Can you work these out from the model? Positions are in its coordinate system, mm. A direction names the side the tool comes from. Give positions to 0.01 mm unless a question says otherwise; leave off trailing zeros. Write each loop counter-clockwise with the first axis right and the second up, starting at its lowest first coordinate (ties: lowest second). Pieces come first, ordered by that corner, then holes. Notation, with made-up numbers: (5, 66.5) -> (58, 66.5) arc R24 ccw to (58, 92.5) -> close; hole circle Ø7 at (32, 82). An arc over 180 degrees is marked (long way). Answer as CSV lines item,"result". Start each with the question number.
1. If we section it at D-D on x = -8.5: Write out the boundary of the cut face in (y, z), plus the area to 3 significant figures.
2. I need wall thicknesses on line 1 (Z direction, x = -25.5, y = 0); line 2 (Z direction, x = 3.5, y = 0); line 3 (X direction, y = -1, z = -8). Which ranges of each line are inside material? Lowest first, please. Write a range as [from, to].
3. On a 3-axis mill with a long thin cutter (end or side, diameter ignored), from which of +Z, -Z, +X, -X, +Y, -Y can I reach the whole of each face in a straight line? I mean faces 1 (the face through (15.1, -1.5, 11.4)), 2 (the face through (-24.93, -4.38, -8.43)), 3 (the face through (0.1, 12.5, -0.1)). Say none if no direction works.
4. If we section it at C-C on x = 1: Write out the boundary of the cut face in (y, z), plus the area to 3 significant figures.
5. I'm going to push flat-ended pins straight in: P1, Ø3, axis at x = 11, z = 3.5, coming from the -Y side; P2, Ø12, axis at y = 0, z = 0, coming from the -X side; P3, Ø5, axis at x = 13.5, z = 9, coming from the -Y side; P4, Ø3, axis at x = -16.5, z = -3, coming from the +Y side. Where does each tip first touch, or does it pass through?
6. If we section it at B-B on y = 0: Write out the boundary of the cut face in (x, z), plus the area to 3 significant figures.
7. If we mould it in two halves opening along Y, with no side actions, what happens to faces 4 (the face through (10, -5, -11)), 5 (the face through (0.1, -12.5, 0.1)), 6 (the face through (0.14, 12.534, -7.29)), 7 (the face through (0.1, 0, 14.5))? For each: pulls with the +Y half, pulls with the -Y half, needs draft (parallel to the pull), parting line crosses it, or undercut.
8. If we section it at A-A on z = 0: Write out the boundary of the cut face in (x, y).
```python
from build123d import *

# Parameters (mm, degrees)
F0_R     = 8.5
F1_DEPTH = 10
F2_R     = 11.5
F2_R_2   = 8.5
F3_DEPTH = 20
F4_R     = 9.5
F4_R_2   = 7.5
F5_DEPTH = 10
F6_R     = 9.5
F7_DEPTH = 25


with BuildPart() as f1:
    # F0 (on Right) → F1 (new body, symmetric)
    with BuildSketch(Plane.YZ):
        with BuildLine():
            ThreePointArc((11.6835483463, -4.4435006516), (12.2941928228, -2.2589428581), (12.5, 0))
            ThreePointArc((12.5, 0), (12.2941928228, 2.2589428581), (11.6835483463, 4.4435006516))
            ThreePointArc((11.6835483463, 4.4435006516), (10.8253175473, 6.25), (9.6899586191, 7.8964993484))
            ThreePointArc((9.6899586191, 7.8964993484), (6.25, 10.8253175473), (1.9935897271, 12.34))
            ThreePointArc((1.9935897271, 12.34), (0, 12.5), (-1.9935897271, 12.34))
            ThreePointArc((-1.9935897271, 12.34), (-6.25, 10.8253175473), (-9.6899586191, 7.8964993484))
            ThreePointArc((-9.6899586191, 7.8964993484), (-10.8253175473, 6.25), (-11.6835483463, 4.4435006516))
            ThreePointArc((-11.6835483463, 4.4435006516), (-12.5, 0), (-11.6835483463, -4.4435006516))
            ThreePointArc((-11.6835483463, -4.4435006516), (-10.8253175473, -6.25), (-9.6899586191, -7.8964993484))
            ThreePointArc((-9.6899586191, -7.8964993484), (-6.25, -10.8253175473), (-1.9935897271, -12.34))
            ThreePointArc((-1.9935897271, -12.34), (0, -12.5), (1.9935897271, -12.34))
            ThreePointArc((1.9935897271, -12.34), (6.25, -10.8253175473), (9.6899586191, -7.8964993484))
            ThreePointArc((9.6899586191, -7.8964993484), (10.8253175473, -6.25), (11.6835483463, -4.4435006516))
        make_face()
        Circle(F0_R, mode=Mode.SUBTRACT)
        with BuildLine():
            ThreePointArc((9.6899586191, 7.8964993484), (10.8253175473, 6.25), (11.6835483463, 4.4435006516))
            ThreePointArc((11.6835483463, 4.4435006516), (12.5573683549, 7.25), (9.6899586191, 7.8964993484))
        make_face()
        with BuildLine():
            ThreePointArc((9.6899586191, -7.8964993484), (12.5573683549, -7.25), (11.6835483463, -4.4435006516))
            ThreePointArc((11.6835483463, -4.4435006516), (10.8253175473, -6.25), (9.6899586191, -7.8964993484))
        make_face()
        with BuildLine():
            ThreePointArc((-1.9935897271, 12.34), (0, 12.5), (1.9935897271, 12.34))
            ThreePointArc((1.9935897271, 12.34), (0, 14.5), (-1.9935897271, 12.34))
        make_face()
        with BuildLine():
            ThreePointArc((-1.9935897271, -12.34), (0, -14.5), (1.9935897271, -12.34))
            ThreePointArc((1.9935897271, -12.34), (0, -12.5), (-1.9935897271, -12.34))
        make_face()
        with BuildLine():
            ThreePointArc((-11.6835483463, 4.4435006516), (-10.8253175473, 6.25), (-9.6899586191, 7.8964993484))
            ThreePointArc((-9.6899586191, 7.8964993484), (-12.5573683549, 7.25), (-11.6835483463, 4.4435006516))
        make_face()
        with BuildLine():
            ThreePointArc((-11.6835483463, -4.4435006516), (-12.5573683549, -7.25), (-9.6899586191, -7.8964993484))
            ThreePointArc((-9.6899586191, -7.8964993484), (-10.8253175473, -6.25), (-11.6835483463, -4.4435006516))
        make_face()
    extrude(amount=F1_DEPTH, both=True)

    # F2 (on Right) → F3 (join, symmetric)
    with BuildSketch(Plane.YZ):
        Circle(F2_R)
        Circle(F2_R_2, mode=Mode.SUBTRACT)
    extrude(amount=F3_DEPTH, both=True)

    # F4 (on face) → F5 (join)
    with BuildSketch(Plane(origin=(-20, 0, 0), x_dir=(0, -1, 0), z_dir=(-1, 0, 0))):
        Circle(F4_R)
        Circle(F4_R_2, mode=Mode.SUBTRACT)
    extrude(amount=F5_DEPTH)

    # F6 (on face) → F7 (cut)
    with BuildSketch(Plane.YZ.offset(20)):
        Circle(F6_R)
    extrude(amount=-F7_DEPTH, mode=Mode.SUBTRACT)


solid = f1.part
```
Computed values:
1,outline,"(-11.68, -4.44) arc R2 ccw (long way) to (-9.69, -7.9) arc R12.5 ccw to (-1.99, -12.34) arc R2 ccw (long way) to (1.99, -12.34) arc R12.5 ccw to (9.69, -7.9) arc R2 ccw (long way) to (11.68, -4.44) arc R12.5 ccw to (11.68, 4.44) arc R2 ccw (long way) to (9.69, 7.9) arc R12.5 ccw to (1.99, 12.34) arc R2 ccw (long way) to (-1.99, 12.34) arc R12.5 ccw to (-9.69, 7.9) arc R2 ccw (long way) to (-11.68, 4.44) arc R12.5 ccw to start; hole circle Ø17 at (0, 0)"
1,area,"303 mm2"
2,line 1,"z = [-9.5, -7.5], [7.5, 9.5]"
2,line 2,"z = [-14.5, -9.5], [9.5, 14.5]"
2,line 3,"x = [-30, -20]"
3,face 1,"+X"
3,face 2,"-X"
3,face 3,"+X, -X, +Y"
4,outline,"(-11.68, -4.44) arc R2 ccw (long way) to (-9.69, -7.9) arc R12.5 ccw to (-1.99, -12.34) arc R2 ccw (long way) to (1.99, -12.34) arc R12.5 ccw to (9.69, -7.9) arc R2 ccw (long way) to (11.68, -4.44) arc R12.5 ccw to (11.68, 4.44) arc R2 ccw (long way) to (9.69, 7.9) arc R12.5 ccw to (1.99, 12.34) arc R2 ccw (long way) to (-1.99, 12.34) arc R12.5 ccw to (-9.69, 7.9) arc R2 ccw (long way) to (-11.68, 4.44) arc R12.5 ccw to start; hole circle Ø19 at (0, 0)"
4,area,"246 mm2"
5,P1,"stops at y = -12.27"
5,P2,"passes through"
5,P3,"stops at y = -9.49"
5,P4,"stops at y = 11.4"
6,outline,"(-30, -9.5) -> (-20, -9.5) -> (-20, -11.5) -> (-10, -11.5) -> (-10, -14.5) -> (10, -14.5) -> (10, -11.5) -> (20, -11.5) -> (20, -9.5) -> (-5, -9.5) -> (-5, -8.5) -> (-20, -8.5) -> (-20, -7.5) -> (-30, -7.5) -> close; (-30, 7.5) -> (-20, 7.5) -> (-20, 8.5) -> (-5, 8.5) -> (-5, 9.5) -> (20, 9.5) -> (20, 11.5) -> (10, 11.5) -> (10, 14.5) -> (-10, 14.5) -> (-10, 11.5) -> (-20, 11.5) -> (-20, 9.5) -> (-30, 9.5) -> close"
6,area,"350 mm2"
7,face 4,"needs draft"
7,face 5,"pulls with the -Y half"
7,face 6,"undercut"
7,face 7,"parting line crosses it"
8,outline,"(-30, -9.5) -> (-20, -9.5) -> (-20, -11.5) -> (-10, -11.5) -> (-10, -12.5) -> (10, -12.5) -> (10, -11.5) -> (20, -11.5) -> (20, -9.5) -> (-5, -9.5) -> (-5, -8.5) -> (-20, -8.5) -> (-20, -7.5) -> (-30, -7.5) -> close; (-30, 7.5) -> (-20, 7.5) -> (-20, 8.5) -> (-5, 8.5) -> (-5, 9.5) -> (20, 9.5) -> (20, 11.5) -> (10, 11.5) -> (10, 12.5) -> (-10, 12.5) -> (-10, 11.5) -> (-20, 11.5) -> (-20, 9.5) -> (-30, 9.5) -> close"
